For this review, take the finished solid that the model builds, in its own axes (mm). Coordinates: 2 decimals unless noted, no trailing zeros. Write each loop counter-clockwise with the first axis right and the second up, starting at its lowest first coordinate (ties: lowest second). Pieces come first, ordered by that corner, then holes.
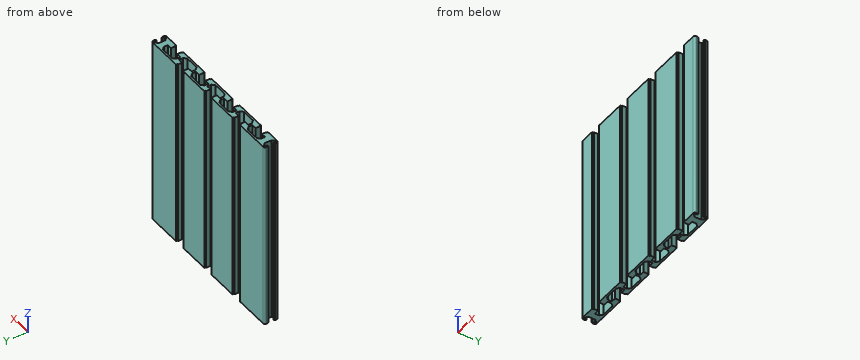
```python
from build123d import *

# Parameters (mm, degrees)
EXTRUDE_1_DEPTH = 200


with BuildPart() as part:
    # Эскиз1 → Бобышка-Вытянуть1 (new body)
    with BuildSketch(Plane.XY):
        with BuildLine():
            Line((-85.853717104, -6.166822364), (-87.303717104, -6.166822364))
            Line((-87.303717104, -6.166822364), (-87.303717104, -3.166822364))
            Line((-87.303717104, -3.166822364), (-88.303717104, -3.166822364))
            Line((-88.303717104, -3.166822364), (-88.303717104, -3.666822364))
            Line((-88.303717104, -3.666822364), (-88.803717104, -3.666822364))
            Line((-88.803717104, -3.666822364), (-88.803717104, -5.666822356))
            ThreePointArc((-88.803717104, -5.666822356), (-88.217930664, -7.081035924), (-86.803717096, -7.666822364))
            Line((-86.803717096, -7.666822364), (-72.103717104, -7.666822364))
            Line((-72.103717104, -7.666822364), (-72.103717104, -6.166822364))
            Line((-72.103717104, -6.166822364), (-71.303717104, -6.166822364))
            Line((-71.303717104, -6.166822364), (-71.303717104, -1.666822364))
            Line((-71.303717104, -1.666822364), (-76.353717104, -1.666822364))
            Line((-76.353717104, -1.666822364), (-76.353717104, 2.533177636))
            Line((-76.353717104, 2.533177636), (-73.553717104, 5.333177636))
            Line((-73.553717104, 5.333177636), (-59.053717104, 5.333177636))
            Line((-59.053717104, 5.333177636), (-56.253717104, 2.533177636))
            Line((-56.253717104, 2.533177636), (-56.253717104, -1.666822364))
            Line((-56.253717104, -1.666822364), (-61.303717104, -1.666822364))
            Line((-61.303717104, -1.666822364), (-61.303717104, -6.166822364))
            Line((-61.303717104, -6.166822364), (-60.503717104, -6.166822364))
            Line((-60.503717104, -6.166822364), (-60.503717104, -7.666822364))
            Line((-60.503717104, -7.666822364), (-27.103717104, -7.666822364))
            Line((-27.103717104, -7.666822364), (-27.103717104, -6.166822364))
            Line((-27.103717104, -6.166822364), (-26.303717104, -6.166822364))
            Line((-26.303717104, -6.166822364), (-26.303717104, -1.666822364))
            Line((-26.303717104, -1.666822364), (-31.353717104, -1.666822364))
            Line((-31.353717104, -1.666822364), (-31.353717104, 2.533177636))
            Line((-31.353717104, 2.533177636), (-28.553717104, 5.333177636))
            Line((-28.553717104, 5.333177636), (-14.053717104, 5.333177636))
            Line((-14.053717104, 5.333177636), (-11.253717104, 2.533177636))
            Line((-11.253717104, 2.533177636), (-11.253717104, -1.666822364))
            Line((-11.253717104, -1.666822364), (-16.303717104, -1.666822364))
            Line((-16.303717104, -1.666822364), (-16.303717104, -6.166822364))
            Line((-16.303717104, -6.166822364), (-15.503717104, -6.166822364))
            Line((-15.503717104, -6.166822364), (-15.503717104, -7.666822364))
            Line((-15.503717104, -7.666822364), (17.896282896, -7.666822364))
            Line((17.896282896, -7.666822364), (17.896282896, -6.166822364))
            Line((17.896282896, -6.166822364), (18.696282896, -6.166822364))
            Line((18.696282896, -6.166822364), (18.696282896, -1.666822364))
            Line((18.696282896, -1.666822364), (13.646282896, -1.666822364))
            Line((13.646282896, -1.666822364), (13.646282896, 2.533177636))
            Line((13.646282896, 2.533177636), (16.446282896, 5.333177636))
            Line((16.446282896, 5.333177636), (30.946282896, 5.333177636))
            Line((30.946282896, 5.333177636), (33.746282896, 2.533177636))
            Line((33.746282896, 2.533177636), (33.746282896, -1.666822364))
            Line((33.746282896, -1.666822364), (28.696282896, -1.666822364))
            Line((28.696282896, -1.666822364), (28.696282896, -6.166822364))
            Line((28.696282896, -6.166822364), (29.496282896, -6.166822364))
            Line((29.496282896, -6.166822364), (29.496282896, -7.666822364))
            Line((29.496282896, -7.666822364), (62.896282896, -7.666822364))
            Line((62.896282896, -7.666822364), (62.896282896, -6.166822364))
            Line((62.896282896, -6.166822364), (63.696282896, -6.166822364))
            Line((63.696282896, -6.166822364), (63.696282896, -1.666822364))
            Line((63.696282896, -1.666822364), (58.646282896, -1.666822364))
            Line((58.646282896, -1.666822364), (58.646282896, 2.533177636))
            Line((58.646282896, 2.533177636), (61.446282896, 5.333177636))
            Line((61.446282896, 5.333177636), (75.946282896, 5.333177636))
            Line((75.946282896, 5.333177636), (78.746282896, 2.533177636))
            Line((78.746282896, 2.533177636), (78.746282896, -1.666822364))
            Line((78.746282896, -1.666822364), (73.696282896, -1.666822364))
            Line((73.696282896, -1.666822364), (73.696282896, -6.166822364))
            Line((73.696282896, -6.166822364), (74.496282896, -6.166822364))
            Line((74.496282896, -6.166822364), (74.496282896, -7.666822364))
            Line((74.496282896, -7.666822364), (89.196282888, -7.666822364))
            ThreePointArc((89.196282888, -7.666822364), (90.610496456, -7.081035924), (91.196282896, -5.666822356))
            Line((91.196282896, -5.666822356), (91.196282896, -3.666822364))
            Line((91.196282896, -3.666822364), (90.696282896, -3.666822364))
            Line((90.696282896, -3.666822364), (90.696282896, -3.166822364))
            Line((90.696282896, -3.166822364), (89.696282896, -3.166822364))
            Line((89.696282896, -3.166822364), (89.696282896, -6.166822364))
            Line((89.696282896, -6.166822364), (88.246282896, -6.166822364))
            Line((88.246282896, -6.166822364), (85.696282896, -3.616822364))
            Line((85.696282896, -3.616822364), (85.696282896, 3.283177636))
            Line((85.696282896, 3.283177636), (88.246282896, 5.833177636))
            Line((88.246282896, 5.833177636), (89.696282896, 5.833177636))
            Line((89.696282896, 5.833177636), (89.696282896, 2.833177636))
            Line((89.696282896, 2.833177636), (90.696282896, 2.833177636))
            Line((90.696282896, 2.833177636), (90.696282896, 3.333177636))
            Line((90.696282896, 3.333177636), (91.196282896, 3.333177636))
            Line((91.196282896, 3.333177636), (91.196282896, 5.333177628))
            ThreePointArc((91.196282896, 5.333177628), (90.610496456, 6.747391196), (89.196282888, 7.333177636))
            Line((89.196282888, 7.333177636), (51.996282896, 7.333177636))
            Line((51.996282896, 7.333177636), (51.996282896, 5.833177636))
            Line((51.996282896, 5.833177636), (51.196282898, 5.833177636))
            Line((51.196282898, 5.833177636), (51.196282898, 1.333177634))
            Line((51.196282898, 1.333177634), (56.246282898, 1.333177634))
            Line((56.246282898, 1.333177634), (56.246282898, -2.866822366))
            Line((56.246282898, -2.866822366), (53.446282898, -5.666822366))
            Line((53.446282898, -5.666822366), (38.946282898, -5.666822366))
            Line((38.946282898, -5.666822366), (36.146282898, -2.866822366))
            Line((36.146282898, -2.866822366), (36.146282898, 1.333177634))
            Line((36.146282898, 1.333177634), (41.196282898, 1.333177634))
            Line((41.196282898, 1.333177634), (41.196282898, 5.833177636))
            Line((41.196282898, 5.833177636), (40.396282896, 5.833177636))
            Line((40.396282896, 5.833177636), (40.396282896, 7.333177636))
            Line((40.396282896, 7.333177636), (6.996282896, 7.333177636))
            Line((6.996282896, 7.333177636), (6.996282896, 5.833177636))
            Line((6.996282896, 5.833177636), (6.196282898, 5.833177636))
            Line((6.196282898, 5.833177636), (6.196282898, 1.333177634))
            Line((6.196282898, 1.333177634), (11.246282898, 1.333177634))
            Line((11.246282898, 1.333177634), (11.246282898, -2.866822366))
            Line((11.246282898, -2.866822366), (8.446282898, -5.666822366))
            Line((8.446282898, -5.666822366), (-6.053717102, -5.666822366))
            Line((-6.053717102, -5.666822366), (-8.853717102, -2.866822366))
            Line((-8.853717102, -2.866822366), (-8.853717102, 1.333177634))
            Line((-8.853717102, 1.333177634), (-3.803717102, 1.333177634))
            Line((-3.803717102, 1.333177634), (-3.803717102, 5.833177636))
            Line((-3.803717102, 5.833177636), (-4.603717104, 5.833177636))
            Line((-4.603717104, 5.833177636), (-4.603717104, 7.333177636))
            Line((-4.603717104, 7.333177636), (-38.003717104, 7.333177636))
            Line((-38.003717104, 7.333177636), (-38.003717104, 5.833177636))
            Line((-38.003717104, 5.833177636), (-38.803717102, 5.833177636))
            Line((-38.803717102, 5.833177636), (-38.803717102, 1.333177634))
            Line((-38.803717102, 1.333177634), (-33.753717102, 1.333177634))
            Line((-33.753717102, 1.333177634), (-33.753717102, -2.866822366))
            Line((-33.753717102, -2.866822366), (-36.553717102, -5.666822366))
            Line((-36.553717102, -5.666822366), (-51.053717102, -5.666822366))
            Line((-51.053717102, -5.666822366), (-53.853717102, -2.866822366))
            Line((-53.853717102, -2.866822366), (-53.853717102, 1.333177634))
            Line((-53.853717102, 1.333177634), (-48.803717102, 1.333177634))
            Line((-48.803717102, 1.333177634), (-48.803717102, 5.833177636))
            Line((-48.803717102, 5.833177636), (-49.603717104, 5.833177636))
            Line((-49.603717104, 5.833177636), (-49.603717104, 7.333177636))
            Line((-49.603717104, 7.333177636), (-86.803717096, 7.333177636))
            ThreePointArc((-86.803717096, 7.333177636), (-88.217930664, 6.747391196), (-88.803717104, 5.333177628))
            Line((-88.803717104, 5.333177628), (-88.803717104, 3.333177636))
            Line((-88.803717104, 3.333177636), (-88.303717104, 3.333177636))
            Line((-88.303717104, 3.333177636), (-88.303717104, 2.833177636))
            Line((-88.303717104, 2.833177636), (-87.303717104, 2.833177636))
            Line((-87.303717104, 2.833177636), (-87.303717104, 5.833177636))
            Line((-87.303717104, 5.833177636), (-85.853717104, 5.833177636))
            Line((-85.853717104, 5.833177636), (-83.303717104, 3.283177636))
            Line((-83.303717104, 3.283177636), (-83.303717104, -3.616822364))
            Line((-83.303717104, -3.616822364), (-85.853717104, -6.166822364))
        make_face()
    extrude(amount=EXTRUDE_1_DEPTH)


solid = part.part
```
Q1. Add section A-A (x = -23). State the section outline as (y, z) points.
Ans:
outline: (5.33, 0) - (7.33, 0) - (7.33, 200) - (5.33, 200) - close
Q2. Clearance check with flat-ended pins moving along their axes: pin 1 Ø6 at (x, z) = (24, 130.5) entering from -Y; pin 2 Ø1.1 at (x, z) = (90, 60) entering from +Y; pin 3 Ø0.9 at (x, z) = (41, 88) entering from +Y. State where each tip first meets the part, or that it passes through.
Ans:
pin 1: stops at y = 5.33
pin 2: stops at y = 7.32
pin 3: stops at y = 5.83
Q3. For probe 1 along Y at (x, z) = (78, 34); probe 2 along Y at (x, z) = (-37, 141); probe 3 along X at (y, z) = (6.75, 30), list the stretches that pass through material, from the lowest coordinate up.
Ans:
probe 1: y = -7.67 to -1.67, 3.28 to 7.33
probe 2: y = -7.67 to -5.67, 1.33 to 7.33
probe 3: x = -88.22 to -49.6, -38 to -4.6, 7 to 40.4, 52 to 90.61
